Geometry check sheet. Reference: the model listing, model coordinates, mm. A direction names the side the tool comes from. Coordinates: 2 decimals unless noted, no trailing zeros.
from build123d import *

# Parameters (mm, degrees)
SKETCH002_R     = 50
SKETCH002_R_2   = 2.15
SKETCH002_R_3   = 9
SKETCH002_R_4   = 12
PAD001_DEPTH    = 8
CHAMFER001_SIZE = 1
SKETCH003_R     = 12.7
SKETCH003_R_2   = 9
PAD002_DEPTH    = 8
CHAMFER002_SIZE = 0.5


with BuildPart() as part:
    # Sketch002 → Pad001 (new body)
    with BuildSketch(Plane.XY):
        Circle(SKETCH002_R)
        with Locations((-30.479838, 30.479838)):
            Circle(SKETCH002_R_2, mode=Mode.SUBTRACT)
        with Locations((30.479838, 30.479838)):
            Circle(SKETCH002_R_2, mode=Mode.SUBTRACT)
        with Locations((30.479838, -30.479838)):
            Circle(SKETCH002_R_2, mode=Mode.SUBTRACT)
        with Locations((-30.479838, -30.479838)):
            Circle(SKETCH002_R_2, mode=Mode.SUBTRACT)
        Circle(SKETCH002_R_3, mode=Mode.SUBTRACT)
        with Locations((-30.479838, 0)):
            Circle(SKETCH002_R_4, mode=Mode.SUBTRACT)
        with Locations((30.479838, 0)):
            Circle(SKETCH002_R_4, mode=Mode.SUBTRACT)
        with Locations((0, -30.479838)):
            Circle(SKETCH002_R_4, mode=Mode.SUBTRACT)
        with Locations((0, 30.479838)):
            Circle(SKETCH002_R_4, mode=Mode.SUBTRACT)
    extrude(amount=PAD001_DEPTH)

    # Chamfer001
    chamfer001_edges = [part.edges().sort_by_distance(p)[0] for p in [
        (-50, 0, 8),
        (-42.479838, 0, 8),
        (-12, 30.479838, 8),
        (18.479838, 0, 8),
        (-12, -30.479838, 8),
        (-9, 0, 8),
        (-32.629838, -30.479838, 8),
        (28.329838, -30.479838, 8),
        (28.329838, 30.479838, 8),
        (-32.629838, 30.479838, 8),
        (-50, 0, 0),
        (-42.479838, 0, 0),
        (-12, 30.479838, 0),
        (18.479838, 0, 0),
        (-12, -30.479838, 0),
        (-9, 0, 0),
        (-32.629838, -30.479838, 0),
        (28.329838, -30.479838, 0),
        (28.329838, 30.479838, 0),
        (-32.629838, 30.479838, 0),
    ]]
    chamfer(chamfer001_edges, length=CHAMFER001_SIZE)

    # Sketch003 (on Face12 of Pad001) → Pad002 (join)
    with BuildSketch(Plane.XY.offset(6)):
        Circle(SKETCH003_R)
        Circle(SKETCH003_R_2, mode=Mode.SUBTRACT)
    extrude(amount=PAD002_DEPTH)

    # Chamfer002
    chamfer002_edges = [part.edges().sort_by_distance(p)[0] for p in [
        (-12.7, 0, 14),
        (-9, 0, 14),
    ]]
    chamfer(chamfer002_edges, length=CHAMFER002_SIZE)


solid = part.part
1) Material ranges on probe 1 along Y at (x, z) = (29, 1.75); probe 2 along Y at (x, z) = (-29.5, 1.75); probe 3 along X at (y, z) = (-32, 3), recorded low to high.
Data:
probe 1: y = -40.73 to -32.04, -28.92 to -11.91, 11.91 to 28.92, 32.04 to 40.73
probe 2: y = -40.37 to -32.39, -28.57 to -11.96, 11.96 to 28.57, 32.39 to 40.37
probe 3: x = -38.42 to -32, -28.96 to -11.9, 11.9 to 28.96, 32 to 38.42
2) Section check A-A on y = 0. Count the separate pieces of the cut face and the enclosed holes in it, and give its area (3 significant figures).
Data:
separate pieces: 4
enclosed holes: 0
area: 309 mm2
3) Access from +Z, -Z, +X, -X, +Y, -Y to the whole of each face (thin tool, end or side, straight path). Record for faces 4 (the cylindrical face through (-32.064, -29.027, 3.958)), 5 (the flat face through (10, -10, 8)).
Data:
face 4: +Z, -Z
face 5: +Z
4) Mould release check, pull along Y, two halves, no side actions. Record for faces 1 (the cylindrical face through (47.69, 15.02, 3.96)), 2 (the flat face through (0, -10, 14)), 3 (the cylindrical face through (-2.601, 18.765, 3.958)): +Y half, -Y half, draft (parallel to the pull), parting line (faces both ways), or undercut.
Data:
face 1: parting line
face 2: draft
face 3: undercut
5) Depth check by flat-ended pin: pin 1 (4 mm diameter, centred on x = -11.5, y = 24, fed in from +Z); pin 2 (1.5 mm diameter, centred on y = 14, z = 4, fed in from +X); pin 3 (1 mm diameter, centred on y = -31.5, z = 5.5, fed in from +X). Enter the tip coordinate at first touch or a pass-through.
Data:
pin 1: stops at z = 8
pin 2: stops at x = 48.21
pin 3: stops at x = 39.23
